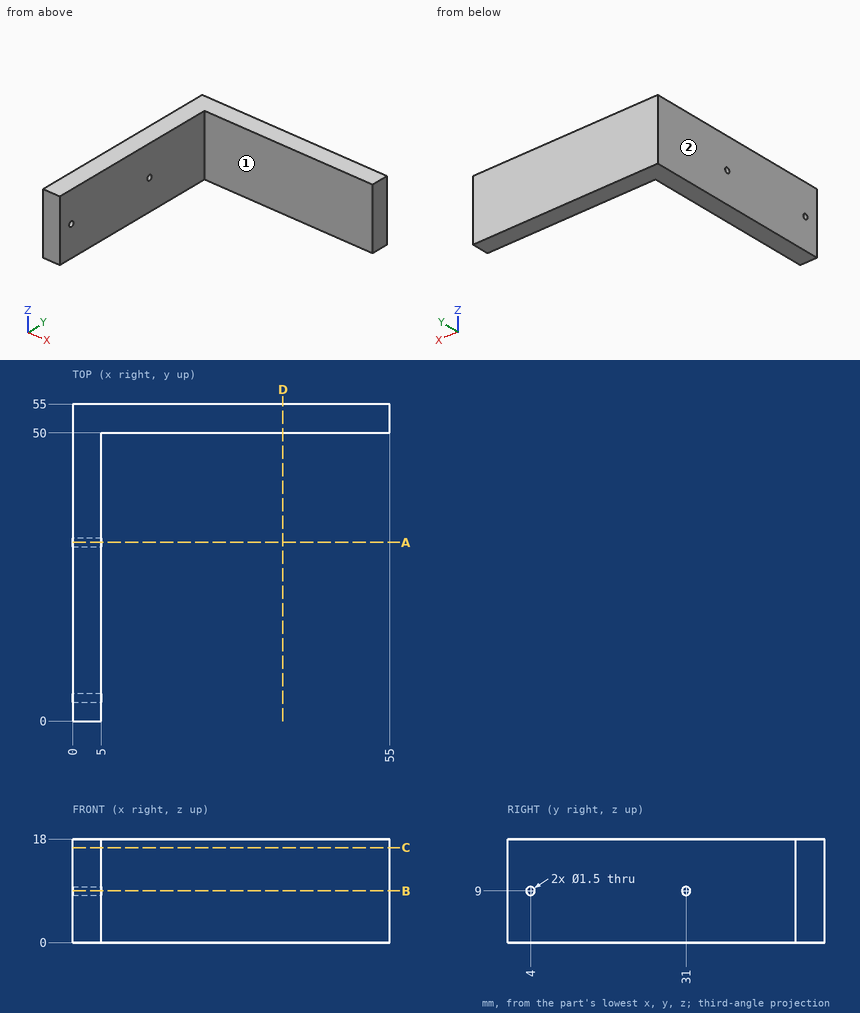
Part print with two shaded views. Sizes in mm from the minimum x, y, z corner. A direction names the side the tool comes from. Give positions to 0.01 mm unless a question says otherwise; leave off trailing zeros. Write each loop counter-clockwise with the first axis right and the second up, starting at its lowest first coordinate (ties: lowest second). Pieces come first, ordered by that corner, then holes.
1) Which spindle directions (+Z, -Z, +X, -X, +Y, -Y) get a long thin tool onto all of the face, cutting with end or side? Do the marked faces 1 and 2. Say none if no direction does.
Resolved:
face 1: +Z, -Z, +X, -Y
face 2: +Z, -Z, -X, +Y, -Y
2) Pin check, flat tips, straight feed: pin 1 (9 mm diameter, centred on x = 39.5, z = 8.5, fed in from -Y); pin 2 (2.5 mm diameter, centred on y = 4, z = 9, fed in from +X). Stop position of each tip, or through.
Resolved:
pin 1: stops at y = 50
pin 2: stops at x = 5
3) Cut at D-D on x = 36.5. Write the cut outline in (y, z), then the cut area to 3 significant figures.
Resolved:
outline: (50, 0) - (55, 0) - (55, 18) - (50, 18) - close
area: 90.0 mm2
4) Probe L1, parallel to Z at x = 2.5, y = 4; L2, parallel to Y at x = 7.5, z = 10.25; L3, parallel to X at y = 43, z = 7.5. List the from-to ranges inside material, lowest first.
Resolved:
L1: z = 0 to 8.25, 9.75 to 18
L2: y = 50 to 55
L3: x = 0 to 5
5) Cut at B-B on z = 9. Write the cut outline in (x, y).
Resolved:
outline: (0, 0) - (5, 0) - (5, 3.25) - (0, 3.25) - close; (0, 4.75) - (5, 4.75) - (5, 30.25) - (0, 30.25) - close; (0, 31.75) - (5, 31.75) - (5, 50) - (55, 50) - (55, 55) - (0, 55) - close
6) Cut at A-A on y = 31. Write the cut outline in (x, z), then the cut area to 3 significant figures.
Resolved:
outline: (0, 0) - (5, 0) - (5, 8.25) - (0, 8.25) - close; (0, 9.75) - (5, 9.75) - (5, 18) - (0, 18) - close
area: 82.5 mm2
7) Cut at C-C on z = 16.5. Write the cut outline in (x, y), then the cut area to 3 significant figures.
Resolved:
outline: (0, 0) - (5, 0) - (5, 50) - (55, 50) - (55, 55) - (0, 55) - close
area: 525 mm2
